```python
from build123d import *

# Parameters (mm, degrees)
SKETCH1_R           = 32
BOSS_EXTRUDE1_DEPTH = 10
SKETCH3_W           = 15
SKETCH3_H           = 15
CUT_EXTRUDE1_DEPTH  = 47.346520905
SKETCH4_W           = 10.5
SKETCH4_H           = 10.5
CUT_EXTRUDE2_DEPTH  = 3


with BuildPart() as part:
    # Sketch1 → Boss-Extrude1 (new body)
    with BuildSketch(Plane(origin=(0, 0, 0), x_dir=(1, 0, 0), z_dir=(0, 1, 0))):
        with Locations(Location((0, 0, 0), (0, 0, 270))):
            Circle(SKETCH1_R)
    extrude(amount=BOSS_EXTRUDE1_DEPTH)

    # Cut-Sweep1: sweep along a path in Sketch1_2
    with BuildLine(Plane(origin=(0, 0, 0), x_dir=(1, 0, 0), z_dir=(0, 1, 0))) as cut_sweep1_path:
        CenterArc((0, 0), 32, 0, 360)
    # Sketch2 → Cut-Sweep1 (sweep, cut)
    with BuildSketch(Plane.XY):
        Polygon((32, 10), (29, 5), (32, 0), align=None)
    sweep(path=cut_sweep1_path.line, mode=Mode.SUBTRACT)

    # Sketch3 → Cut-Extrude1 (cut, through all)
    with BuildSketch(Plane(origin=(0, 10, 0), x_dir=(1, 0, 0), z_dir=(0, 1, 0))):
        Rectangle(SKETCH3_W, SKETCH3_H)
    extrude(amount=-CUT_EXTRUDE1_DEPTH, mode=Mode.SUBTRACT)

    # Sketch4 → Cut-Extrude2 (cut)
    with BuildSketch(Plane.XZ):
        with Locations((0, 12.75)):
            Rectangle(SKETCH4_W, SKETCH4_H)
        with Locations((0, -12.75)):
            Rectangle(SKETCH4_W, SKETCH4_H)
    extrude(amount=-CUT_EXTRUDE2_DEPTH, mode=Mode.SUBTRACT)


solid = part.part
```
The model under review builds one solid part; all positions refer to its coordinate system, in mm. A direction names the side the tool comes from. Give positions to 0.01 mm unless a question says otherwise; leave off trailing zeros. Write each loop counter-clockwise with the first axis right and the second up, starting at its lowest first coordinate (ties: lowest second). Pieces come first, ordered by that corner, then holes. Notation, with made-up numbers: M -33.75,88.25 L 4.25,88.25 A11 cw 4.25,100.25 Z; hole C 31.5,-7.5 d9. An arc over 180 degrees is marked long. Write item = value, one per line. Start each with the question number.
Q1. We need section A-A (z = 0). State the section outline as (x, y) points.
Q2. We need section C-C (y = 9). State the section outline as (x, z) points.
Q3. For line 1 (X direction, y = 7.5, z = -0.5); line 2 (Z direction, x = -5.5, y = 4.75); line 3 (Y direction, x = 3, z = -16), list the stretches that pass through material, from the lowest coordinate up.
Q4. Machinability: for faces 5 (the face through (0, 1, 18)), 6 (the face through (26.923, 5.243, 11.163)), 7 (the face through (8, 10, 0)), 8 (the face through (-7.5, 5, 0)), which of the approach directions +Z, -Z, +X, -X, +Y, -Y give a long, thin tool a straight path to every point of the face, cutting with its end or side? Answer none if there is none.
Q5. Clearance check with flat-ended pins moving along their axes: pin 1 (3.5 mm diameter, centred on x = 0.5, y = 1, fed in from -Z); pin 2 (11.5 mm diameter, centred on x = 0, z = 14, fed in from -Y); pin 3 (1 mm diameter, centred on x = -23, y = 3, fed in from +Z); pin 4 (1 mm diameter, centred on y = 9, z = 20.5, fed in from +X). State where each tip first meets the part, or that it passes through.
Q6. We need section B-B (x = 0). State the section outline as (y, z) points.
Q7. Mouldability with a two-part tool opening along Z and no side actions: class faces 1 (the face through (0, 3, -13)), 2 (the face through (0, 6, 7.5)), 3 (the face through (8, 0, 0)), 4 (the face through (-3.8, 4.687, -28.939)) as released by +Z, released by -Z, zero draft, split by the parting line, or undercut.
Result set:
q1.outline = M -32,0 L -7.5,0 L -7.5,10 L -32,10 L -29,5 Z; M 7.5,0 L 32,0 L 29,5 L 32,10 L 7.5,10 Z
q2.outline = C 0,0 d62.8; hole M -7.5,-7.5 L 7.5,-7.5 L 7.5,7.5 L -7.5,7.5 Z
q3.line_1 = -30.5 to -7.5, 7.5 to 30.5
q3.line_2 = -28.63 to -7.5, 7.5 to 28.63
q3.line_3 = 3 to 10
q4.face_5 = -Y
q4.face_6 = none
q4.face_7 = +Z, -Z, +X, -X, +Y
q4.face_8 = +Y, -Y
q5.pin_1 = -32
q5.pin_2 = 0
q5.pin_3 = 20.3
q5.pin_4 = 24.36
q6.outline = M 0,-32 L 5,-29 L 10,-32 L 10,-7.5 L 3,-7.5 L 3,-18 L 0,-18 Z; M 0,18 L 3,18 L 3,7.5 L 10,7.5 L 10,32 L 5,29 L 0,32 Z
q7.face_1 = undercut
q7.face_2 = undercut
q7.face_3 = zero draft
q7.face_4 = split by the parting line
